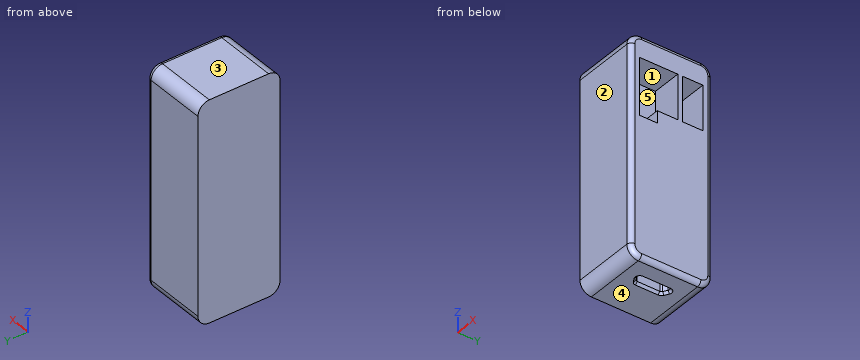
```python
from build123d import *

# Parameters (mm, degrees)
EXTRUDE_1_DEPTH     = 14.6
FILLET_1_R          = 1
CUT_EXTRUDE_1_DEPTH = 8
CHAMFER_1_SIZE      = 0.5
SKETCH_3_W          = 9.8
SKETCH_3_H          = 4.5
CUT_EXTRUDE_2_DEPTH = 6.5


with BuildPart() as part:
    # ｽｹｯﾁ1 → ﾎﾞｽ - 押し出し1 (new body)
    with BuildSketch(Plane(origin=(0, 0, 0), x_dir=(0, 0, -1), z_dir=(1, 0, 0))):
        with BuildLine():
            Line((-21.5, 9), (21.5, 9))
            ThreePointArc((21.5, 9), (23.267766953, 8.267766953), (24, 6.5))
            Line((24, 6.5), (24, -6.5))
            ThreePointArc((24, -6.5), (23.267766953, -8.267766953), (21.5, -9))
            Line((21.5, -9), (-21.5, -9))
            ThreePointArc((-21.5, -9), (-23.267766953, -8.267766953), (-24, -6.5))
            Line((-24, -6.5), (-24, 6.5))
            ThreePointArc((-24, 6.5), (-23.267766953, 8.267766953), (-21.5, 9))
        make_face()
    extrude(amount=EXTRUDE_1_DEPTH)

    # ﾌｨﾚｯﾄ1
    fillet_1_edges = [part.edges().sort_by_distance(p)[0] for p in [
        (14.6, 8.267766953, 23.267766953),
        (14.6, 0, 24),
        (14.6, -8.267766953, 23.267766953),
        (14.6, -9, 0),
        (14.6, -8.267766953, -23.267766953),
        (14.6, 0, -24),
        (14.6, 8.267766953, -23.267766953),
        (14.6, 9, 0),
    ]]
    fillet(fillet_1_edges, radius=FILLET_1_R)

    # ｽｹｯﾁ2 → ｶｯﾄ - 押し出し1 (cut)
    with BuildSketch(Plane(origin=(0, 0, -24), x_dir=(-1, 0, 0), z_dir=(0, 0, -1))):
        with BuildLine():
            Line((-9.15, 3.433012702), (-8.25, 2.91339746))
            ThreePointArc((-8.25, 2.91339746), (-8.066987298, 2.730384758), (-8, 2.480384758))
            Line((-8, 2.480384758), (-8, -2.480384758))
            ThreePointArc((-8, -2.480384758), (-8.066987298, -2.730384758), (-8.25, -2.91339746))
            Line((-8.25, -2.91339746), (-9.15, -3.433012702))
            ThreePointArc((-9.15, -3.433012702), (-9.65, -3.433012702), (-9.9, -3))
            Line((-9.9, -3), (-9.9, 3))
            ThreePointArc((-9.9, 3), (-9.65, 3.433012702), (-9.15, 3.433012702))
        make_face()
    extrude(amount=-CUT_EXTRUDE_1_DEPTH, mode=Mode.SUBTRACT)

    # 面取り1
    chamfer_1_edges = [part.edges().sort_by_distance(p)[0] for p in [
        (8.066987298, -2.730384758, -24),
        (8, 0, -24),
        (8.066987298, 2.730384758, -24),
        (8.7, 3.173205081, -24),
        (9.65, 3.433012702, -24),
        (9.9, 0, -24),
        (9.65, -3.433012702, -24),
        (8.7, -3.173205081, -24),
    ]]
    chamfer(chamfer_1_edges, length=CHAMFER_1_SIZE)

    # ｽｹｯﾁ3 → ｶｯﾄ - 押し出し2 (cut)
    with BuildSketch(Plane(origin=(14.6, 0, 0), x_dir=(0, 0, -1), z_dir=(1, 0, 0))):
        Polygon((-19, 1.425), (-19, -6.925), (-6.55, -6.925), (-6.55, -3.075), (-9.2, -3.075), (-9.2, 1.425), align=None)
        with Locations((-14.1, 4.675)):
            Rectangle(SKETCH_3_W, SKETCH_3_H)
    extrude(amount=-CUT_EXTRUDE_2_DEPTH, mode=Mode.SUBTRACT)


solid = part.part
```
Input: part model. Units: mm. Frame: model coordinates. Face numbers are marked on the shaded views. A direction names the side the tool comes from. Coordinates: 2 decimals unless noted, no trailing zeros. Write each loop counter-clockwise with the first axis right and the second up, starting at its lowest first coordinate (ties: lowest second). Pieces come first, ordered by that corner, then holes.
1) Section B-B on z = 7.5. Output: boundary loops of the cut face in (x, y) (3 decimals), and give its area (3 significant figures).
2) Mould query, pull axis Z, two halves, no side actions, for the marked faces 3, 4 and 5. Classes: pulls with the +Z half, pulls with the -Z half, needs draft (parallel to the pull), parting line crosses it, or undercut.
3) Pin query (flat end, axial travel): pin 1 Ø1.3 at (y, z) = (5.5, 13.5) entering from +X; pin 2 Ø1.5 at (x, y) = (8.5, -1.5) entering from -Z; pin 3 Ø3 at (y, z) = (1.5, -18) entering from -X. Return the tip coordinate at first contact, or that it passes through.
4) Section A-A on x = 11.25. Output: boundary loops of the cut face in (y, z) (3 decimals).
5) Section C-C on y = -6. Output: boundary loops of the cut face in (x, z).
6) Set-up query: the marked faces 1 and 2. Return all of +Z, -Z, +X, -X, +Y, -Y with unobstructed straight access to the full face (end or side cutting, diameter ignored); none if empty.
7) Material intervals for line 1 along Z through (x, y) = (9, 4.75); line 2 along Y through (x, z) = (9.75, 11) (3 decimals); line 3 along Z through (x, y) = (13.5, -4), sorted ascending.
Check result:
1. outline: (0, -9) - (13.6, -9) arc R1 ccw to (14.6, -8) - (14.6, -6.925) - (8.1, -6.925) - (8.1, -3.075) - (14.6, -3.075) - (14.6, 8) arc R1 ccw to (13.6, 9) - (0, 9) - close
1. area: 237 mm2
2. face 3: pulls with the +Z half
2. face 4: pulls with the -Z half
2. face 5: undercut
3. pin 1: stops at x = 8.1
3. pin 2: stops at z = -23.75
3. pin 3: stops at x = 0
4. outline: (-9, -21.5) arc R2.5 ccw to (-6.5, -24) - (6.5, -24) arc R2.5 ccw to (9, -21.5) - (9, 21.5) arc R2.5 ccw to (6.5, 24) - (-6.5, 24) arc R2.5 ccw to (-9, 21.5) - close; hole (-6.925, 6.55) - (-3.075, 6.55) - (-3.075, 9.2) - (1.425, 9.2) - (1.425, 19) - (-6.925, 19) - close; hole (2.425, 9.2) - (6.925, 9.2) - (6.925, 19) - (2.425, 19) - close
5. outline: (0, -24) - (13.6, -24) arc R1 ccw to (14.6, -23) - (14.6, 6.55) - (8.1, 6.55) - (8.1, 19) - (14.6, 19) - (14.6, 23) arc R1 ccw to (13.6, 24) - (0, 24) - close
6. face 1: +X
6. face 2: +Z, -Z, +X, -X, -Y
7. line 1: z = -24 to 9.2, 19 to 24
7. line 2: y = -9 to -6.925, 1.425 to 2.425, 6.925 to 9
7. line 3: z = -24 to 6.55, 19 to 24
